Autodesk Inventor part; units mm, degrees
ref_plane "IP_ball_XY" through (0, 0, 0) normal (1, 0, 0) x (0, 0, -1)
ref_plane "IP_ball_YZ" through (0, 0, 0) normal (0, 0, -1) x (0, 1, 0)
ref_plane "IP_ball_ZX" through (0, 0, 0) normal (0, 1, 0) x (1, 0, 0)
sketch "Sketch_4" plane through (0, 0, 0) normal (0, 0, 1) x (1, 0, 0)
  line L0 (50, 0) -> (-50, 0)
  arc A0 (-2, 3.28) -> (-1.72, 3) centre (-1.72, 3.28) ccw
  line L1 (-1.72, 3) -> (1.72, 3)
  arc A1 (1.72, 3) -> (2, 3.28) centre (1.72, 3.28) ccw
  line L2 (2, 3.28) -> (2, 8)
  arc A2 (2, 8) -> (1.8, 8.2) centre (1.8, 8) ccw
  line L3 (1.8, 8.2) -> (-1.8, 8.2)
  arc A3 (-1.8, 8.2) -> (-2, 8) centre (-1.8, 8) ccw
  line L4 (-2, 8) -> (-2, 3.28)
revolve "Revolution1" add sketch "Sketch_4" angle 360 about axis through (50, 0, 0) along (1, 0, 0)
ref_plane "IP_ball_XY" through (0, 0, 0) normal (1, 0, 0) x (0, 0, -1)
ref_plane "IP_ball_YZ" through (0, 0, 0) normal (0, 0, -1) x (0, 1, 0)
ref_plane "IP_ball_ZX" through (0, 0, 0) normal (0, 1, 0) x (1, 0, 0)
properties part number "110202DT-20-L1260ZZ_ball"
Geometry check sheet. Reference: the model listing, model coordinates, mm. Round coordinates to 2 decimals unless told otherwise and drop trailing zeros. Order: outer loops, then holes, each group sorted by start corner. A loop starts at its lowest first (then second) coordinate and runs counter-clockwise, first axis right, second up. Notation, with made-up numbers: M -36,-30.75 L 19,-30.75 A25 cw 19,0.25 Z; hole C 35.25,16.5 d11. An arc over 180 degrees is marked long. Answer in a Markdown table with one row per item.
(1) Sectioned sample at A-A, the plane y = 0. Record the cut outline in (x, z), and give its area (3 significant figures).
Responses:
| item | result |
|---|---|
| outline | M -2,-8 A0.2 ccw -1.8,-8.2 L 1.8,-8.2 A0.2 ccw 2,-8 L 2,-3.28 A0.28 ccw 1.72,-3 L -1.72,-3 A0.28 ccw -2,-3.28 Z; M -2,3.28 A0.28 ccw -1.72,3 L 1.72,3 A0.28 ccw 2,3.28 L 2,8 A0.2 ccw 1.8,8.2 L -1.8,8.2 A0.2 ccw -2,8 Z |
| area | 41.5 mm² |
(2) Draft check along Z on faces 1 (the face through (0, -3, 0)), 2 (the face through (-2, 3.44, 0.11)), 3 (the face through (-0.03, -1.07, -8.13)). Enter one of: released by +Z, released by -Z, zero draft, split by the parting line, or undercut.
Responses:
| item | result |
|---|---|
| face 1 | undercut |
| face 2 | zero draft |
| face 3 | split by the parting line |
(3) Go/stop test with flat-tipped pins: P1, Ø2, axis at x = 1.5, z = -2.5, coming from the -Y side; P2, Ø1.5, axis at x = 0, y = -2, coming from the +Z side. Record where each tip stops, or that it passes through.
Responses:
| item | result |
|---|---|
| P1 | stops at y = -8.06 |
| P2 | stops at z = 8.1 |
(4) Sectioned sample at C-C, the plane x = 0.7. Record the cut outline in (y, z).
Responses:
| item | result |
|---|---|
| outline | C 0,0 d16.4; hole C 0,0 d6 |
(5) Scan lines: probe 1 along Z at (x, y) = (1.05, 0); probe 2 along Y at (x, z) = (-0.1, -2.5). Record each from-to range of solid material in increasing order. Write a range as from..to.
Responses:
| item | result |
|---|---|
| probe 1 | z = -8.2..-3, 3..8.2 |
| probe 2 | y = -7.81..-1.66, 1.66..7.81 |
